from build123d import *

# Parameters (mm, degrees)
SKETCH_1_W          = 66.5
SKETCH_1_H          = 8.4
EXTRUDE_1_DEPTH     = 13
SKETCH_2_W          = 1.4
SKETCH_2_H          = 2
CUT_EXTRUDE_1_DEPTH = 104
SKETCH_4_R          = 1.5
CUT_EXTRUDE_3_DEPTH = 36.947218251


with BuildPart() as part:
    # 草图1 → 凸台-拉伸1 (new body)
    with BuildSketch(Plane(origin=(0, 0, 0), x_dir=(1, 0, 0), z_dir=(0, 1, 0))):
        Rectangle(SKETCH_1_W, SKETCH_1_H)
    extrude(amount=EXTRUDE_1_DEPTH)

    # 草图2 → 切除-拉伸1 (cut)
    with BuildSketch(Plane(origin=(33.25, 0, 0), x_dir=(0, 0, -1), z_dir=(1, 0, 0))):
        with Locations((-3.5, 9)):
            Rectangle(SKETCH_2_W, SKETCH_2_H)
    extrude(amount=-CUT_EXTRUDE_1_DEPTH, mode=Mode.SUBTRACT)

    # 草图4 → 切除-拉伸3 (cut, through all)
    with BuildSketch(Plane.XZ):
        with Locations(Location((-26, -1.05, 0), (0, 0, 270))):
            Circle(SKETCH_4_R)
        with Locations(Location((-13, -1.05, 0), (0, 0, 270))):
            Circle(SKETCH_4_R)
        with Locations(Location((26, -1.05, 0), (0, 0, 270))):
            Circle(SKETCH_4_R)
        with Locations(Location((13, -1.05, 0), (0, 0, 270))):
            Circle(SKETCH_4_R)
    extrude(amount=-CUT_EXTRUDE_3_DEPTH, mode=Mode.SUBTRACT)


solid = part.part
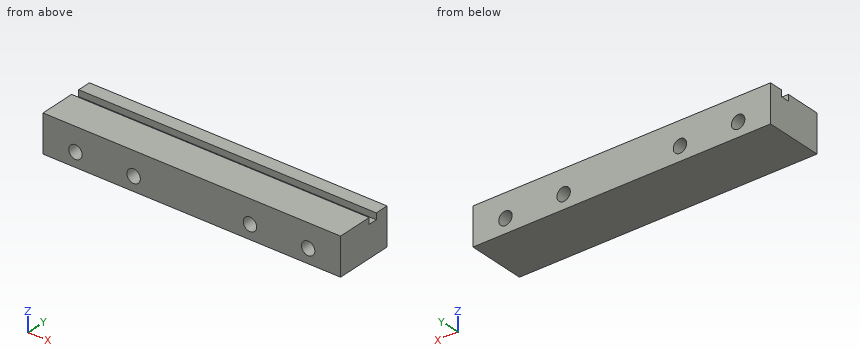
Here's how the part is built. I have some questions about the finished solid (model axes, mm). Coordinates: 2 decimals unless noted, no trailing zeros. Order: outer loops, then holes, each group sorted by start corner. A loop starts at its lowest first (then second) coordinate and runs counter-clockwise, first axis right, second up.
Item 1: If we section it at A-A on z = -1.05: List the corners of the cut face in (x, y) for me.
Result sheet:
outline: (-33.25, 0) - (-27.5, 0) - (-27.5, 13) - (-33.25, 13) - close; (-24.5, 0) - (-14.5, 0) - (-14.5, 13) - (-24.5, 13) - close; (-11.5, 0) - (11.5, 0) - (11.5, 13) - (-11.5, 13) - close; (14.5, 0) - (24.5, 0) - (24.5, 13) - (14.5, 13) - close; (27.5, 0) - (33.25, 0) - (33.25, 13) - (27.5, 13) - close
Item 2: I need wall thicknesses on line 1 (X direction, y = 4.25, z = -1.05); line 2 (Y direction, x = -1.5, z = 3); line 3 (X direction, y = 8.75, z = -2). Which ranges of each line are inside material? Lowest first, please.
Result sheet:
line 1: x = -33.25 to -27.5, -24.5 to -14.5, -11.5 to 11.5, 14.5 to 24.5, 27.5 to 33.25
line 2: y = 0 to 8, 10 to 13
line 3: x = -33.25 to -27.16, -24.84 to -14.16, -11.84 to 11.84, 14.16 to 24.84, 27.16 to 33.25
Item 3: If we section it at C-C on y = 11: List the corners of the cut face in (x, z) for me.
Result sheet:
outline: (-33.25, -4.2) - (33.25, -4.2) - (33.25, 4.2) - (-33.25, 4.2) - close; hole circle Ø3 at (-26, -1.05); hole circle Ø3 at (-13, -1.05); hole circle Ø3 at (13, -1.05); hole circle Ø3 at (26, -1.05)
Item 4: If we section it at D-D on x = -20: List the corners of the cut face in (y, z) for me.
Result sheet:
outline: (0, -4.2) - (13, -4.2) - (13, 4.2) - (10, 4.2) - (10, 2.8) - (8, 2.8) - (8, 4.2) - (0, 4.2) - close
Item 5: If we section it at B-B on x = -13: List the corners of the cut face in (y, z) for me, plus the area to 3 significant figures.
Result sheet:
outline: (0, -4.2) - (13, -4.2) - (13, -2.55) - (0, -2.55) - close; (0, 0.45) - (13, 0.45) - (13, 4.2) - (10, 4.2) - (10, 2.8) - (8, 2.8) - (8, 4.2) - (0, 4.2) - close
area: 67.4 mm2
Item 6: For P1, Ø1.8, axis at x = -26, z = -1.05, coming from the -Y side, with a flat end and sliding along its axis, tell me the tip position at first contact or that it passes through.
Result sheet:
P1: passes through
